Build history of the part. All positions in model axes, mm. A direction names the side the tool comes from. Round coordinates to 2 decimals unless told otherwise and drop trailing zeros. Order: outer loops, then holes, each group sorted by start corner. A loop starts at its lowest first (then second) coordinate and runs counter-clockwise, first axis right, second up. Notation, with made-up numbers: (43, 3.25) -> (73, 3.25) arc R14 cw to (73, 20.25) -> close; hole circle Ø5 at (10.5, -9.75). An arc over 180 degrees is marked (long way). Use a Markdown table: item, result. Add a question column.
Item 1: 3-axis set-ups, long thin cutter, end or side, ignore diameter. For faces 1 (the face through (-11.24, -14.693, 39.549)), 2 (the face through (-27.5, -20, -39)), 3 (the face through (27.5, -20, -39)): which of +Z, -Z, +X, -X, +Y, -Y reach the whole face in a straight line?
Item 2: Two-plate mould, pull along Z, no slides. Class faces 4 (the face through (5, 3.5, 1.6)), 5 (the face through (12, -37, 43)), 6 (the face through (6, 0, 1)), 7 (the face through (-30, 3, -1)): released by +Z, released by -Z, zero draft, split by the parting line, or undercut.
Item 3: Slice it at C-C, the plane x = -2.5. State how many separate pieces and enclosed holes the cut face has, plus the area to 3 significant figures.
Item 4: Probe L1, parallel to Z at x = 0, y = 5.5; L2, parallel to Z at x = -8, y = -43; L3, parallel to X at y = 1.5, z = 0.5. List the from-to ranges inside material, lowest first.
Item 5: Pin check, flat tips, straight feed: pin 1 (2 mm diameter, centred on y = -18.5, z = 38, fed in from +X); pin 2 (2 mm diameter, centred on y = -12, z = -39.5, fed in from -X); pin 3 (1.5 mm diameter, centred on x = -6, y = -48.5, fed in from -Z). Stop position of each tip, or through.
Item 6: Slice it at D-D, the plane y = -36. Give the cut face in (x, z).
Item 7: Slice it at A-A, the plane z = 0. Give the cut face in (x, y), plus the area to 4 significant figures.
Item 8: Slice it at B-B, the plane y = -25. Give the cut face in (x, z), plus the area to 3 significant figures.
from build123d import *

# Parameters (mm, degrees)
F0_W     = 60
F0_H     = 140
F0_R     = 5.25
F1_DEPTH = 7
F2_W     = 60
F2_H     = 7
F3_DEPTH = 27.5
F4_R     = 15.25
F5_DEPTH = 113.001
F6_R     = 20


with BuildPart() as f1:
    # F0 (on Front) → F1 (new body)
    with BuildSketch(Plane.XZ):
        Rectangle(F0_W, F0_H)
        with Locations((0, -60)):
            Circle(F0_R, mode=Mode.SUBTRACT)
        with Locations((0, -30)):
            Circle(F0_R, mode=Mode.SUBTRACT)
        Circle(F0_R, mode=Mode.SUBTRACT)
        with Locations((0, 30)):
            Circle(F0_R, mode=Mode.SUBTRACT)
        with Locations((0, 60)):
            Circle(F0_R, mode=Mode.SUBTRACT)
    extrude(amount=-F1_DEPTH)

    # F2 (on Right) → F3 (join, symmetric)
    with BuildSketch(Plane.YZ):
        with Locations((-30, 39.5)):
            Rectangle(F2_W, F2_H)
        with Locations((-30, -39.5)):
            Rectangle(F2_W, F2_H)
    extrude(amount=F3_DEPTH, both=True)

    # F4 (on face) → F5 (cut, through all)
    with BuildSketch(Plane.XY.offset(43)):
        with Locations((0, -25)):
            Circle(F4_R)
    extrude(amount=-F5_DEPTH, mode=Mode.SUBTRACT)

    # F6
    f6_edges = [f1.edges().sort_by_distance(p)[0] for p in [
        (-30, 3.5, 70),
        (30, 3.5, 70),
        (-27.5, -60, 39.5),
        (27.5, -60, 39.5),
        (-27.5, -60, -39.5),
        (27.5, -60, -39.5),
        (-30, 3.5, -70),
        (30, 3.5, -70),
    ]]
    fillet(f6_edges, radius=F6_R)


solid = f1.part
Check sheet entries:
| question | item | result |
|---|---|---|
| 1 | face 1 | +Z, -Z |
| 1 | face 2 | +Z, -Z, -X, -Y |
| 1 | face 3 | +Z, -Z, +X, -Y |
| 2 | face 4 | undercut |
| 2 | face 5 | released by +Z |
| 2 | face 6 | undercut |
| 2 | face 7 | zero draft |
| 3 | separate pieces | 8 |
| 3 | enclosed holes | 0 |
| 3 | area | 1,080 mm2 |
| 4 | L1 | -70 to -65.25, -54.75 to -35.25, -24.75 to -5.25, 5.25 to 24.75, 35.25 to 54.75, 65.25 to 70 |
| 4 | L2 | -43 to -36, 36 to 43 |
| 4 | L3 | -30 to -5.23, 5.23 to 30 |
| 5 | pin 1 | x = 27.5 |
| 5 | pin 2 | x = -27.5 |
| 5 | pin 3 | z = -43 |
| 6 | outline | (-27.5, -43) -> (-10.56, -43) -> (-10.56, -36) -> (-27.5, -36) -> close; (-27.5, 36) -> (-10.56, 36) -> (-10.56, 43) -> (-27.5, 43) -> close; (10.56, -43) -> (27.5, -43) -> (27.5, -36) -> (10.56, -36) -> close; (10.56, 36) -> (27.5, 36) -> (27.5, 43) -> (10.56, 43) -> close |
| 7 | outline | (-30, 0) -> (-5.25, 0) -> (-5.25, 7) -> (-30, 7) -> close; (5.25, 0) -> (30, 0) -> (30, 7) -> (5.25, 7) -> close |
| 7 | area | 346.5 mm2 |
| 8 | outline | (-27.5, -43) -> (-15.25, -43) -> (-15.25, -36) -> (-27.5, -36) -> close; (-27.5, 36) -> (-15.25, 36) -> (-15.25, 43) -> (-27.5, 43) -> close; (15.25, -43) -> (27.5, -43) -> (27.5, -36) -> (15.25, -36) -> close; (15.25, 36) -> (27.5, 36) -> (27.5, 43) -> (15.25, 43) -> close |
| 8 | area | 343 mm2 |
